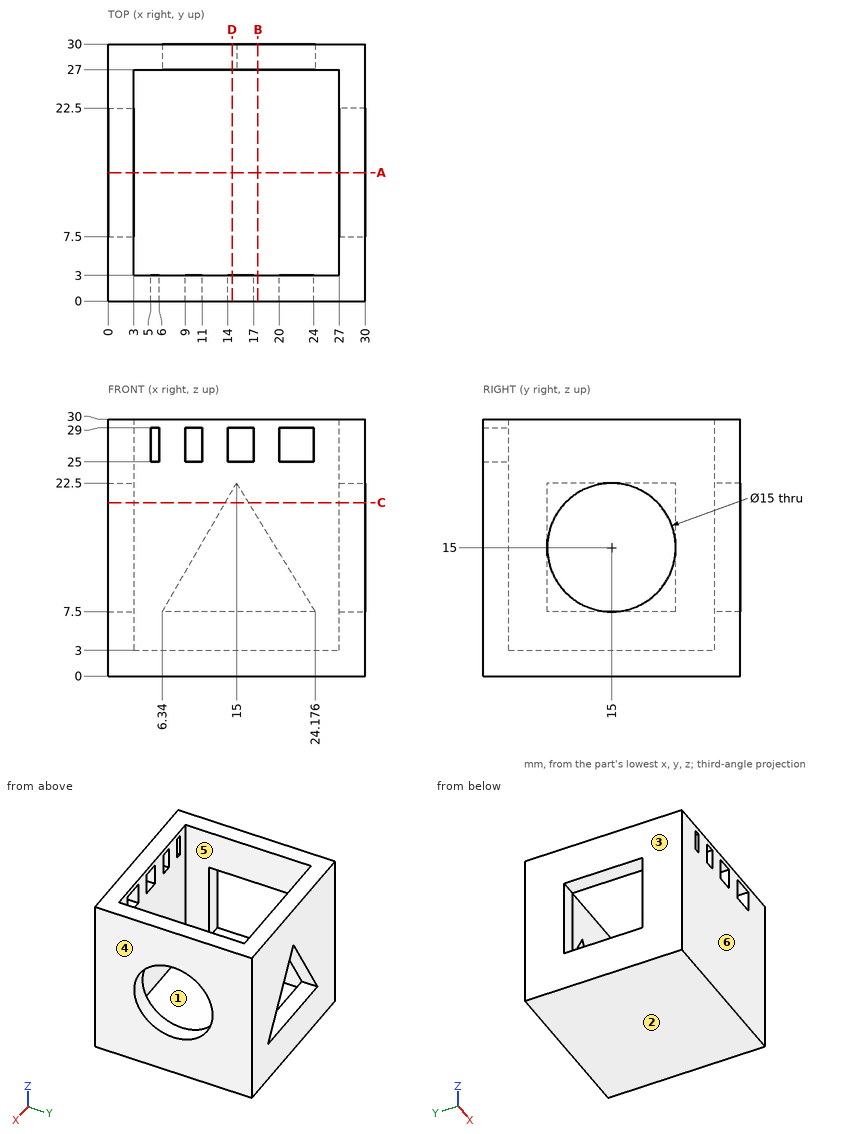
Design review of the part shown in the three views and the two pictorial views. Dimensions are in mm from the part's minimum x, y and z. A direction names the side the tool comes from. Give positions to 0.01 mm unless a question says otherwise; leave off trailing zeros. Write each loop counter-clockwise with the first axis right and the second up, starting at its lowest first coordinate (ties: lowest second). Pieces come first, ordered by that corner, then holes. Notation, with made-up numbers: M 8.25,23.5 L 65.25,23.5 A17 ccw 65.25,56.5 Z; hole C 20,34.25 d11. An arc over 180 degrees is marked long. Return JSON: item names as keys, results as strings. Group by question number.
Item 1: Wall thickness on line 1 along Y through (x, z) = (22.25, 14.5); line 2 along Z through (x, y) = (28.85, 15): over which ranges is each line inside the solid? List them lowest first.
Item 2: The part is to be moulded in two halves that separate along X. For the marked faces 1, 2, 3 and 4, say which applies: pulls with the +X half, pulls with the -X half, needs draft (parallel to the pull), parting line crosses it, or undercut.
Item 3: Take a section at C-C (z = 20.25). Give the boundary of the cut face in (x, y).
Item 4: Take a section at B-B (x = 17.5). Give the boundary of the cut face in (y, z).
Item 5: Tool access review of the marked faces 5 and 6: name each direction out of +Z, -Z, +X, -X, +Y, -Y from which nothing blocks a thin tool from reaching the whole face with its end or side.
Item 6: Take a section at D-D (x = 14.5). Give the boundary of the cut face in (y, z).
Item 7: Take a section at A-A (y = 15). Give the boundary of the cut face in (x, z).
Return value:
{
 "1": {"line 1": "y = 0 to 3, 27 to 30", "line 2": "z = 0 to 7.5, 22.5 to 30"},
 "2": {"face 1": "undercut", "face 2": "needs draft", "face 3": "pulls with the -X half", "face 4": "pulls with the +X half"},
 "3": {"outline": "M 0,0 L 30,0 L 30,9.64 L 27,9.64 L 27,3 L 3,3 L 3,7.5 L 0,7.5 Z; M 0,22.5 L 3,22.5 L 3,27 L 13.7,27 L 13.7,30 L 0,30 Z; M 16.38,27 L 27,27 L 27,20.36 L 30,20.36 L 30,30 L 16.38,30 Z"},
 "4": {"outline": "M 0,0 L 30,0 L 30,7.5 L 27,7.5 L 27,3 L 3,3 L 3,30 L 0,30 Z; M 27,18.41 L 30,18.41 L 30,30 L 27,30 Z"},
 "5": {"face 5": "+Z", "face 6": "+Z, -Z, +X, -X, -Y"},
 "6": {"outline": "M 0,0 L 30,0 L 30,7.5 L 27,7.5 L 27,3 L 3,3 L 3,25 L 0,25 Z; M 0,29 L 3,29 L 3,30 L 0,30 Z; M 27,21.63 L 30,21.63 L 30,30 L 27,30 Z"},
 "7": {"outline": "M 0,0 L 30,0 L 30,7.5 L 27,7.5 L 27,3 L 3,3 L 3,7.5 L 0,7.5 Z; M 0,22.5 L 3,22.5 L 3,30 L 0,30 Z; M 27,22.5 L 30,22.5 L 30,30 L 27,30 Z"}
}
